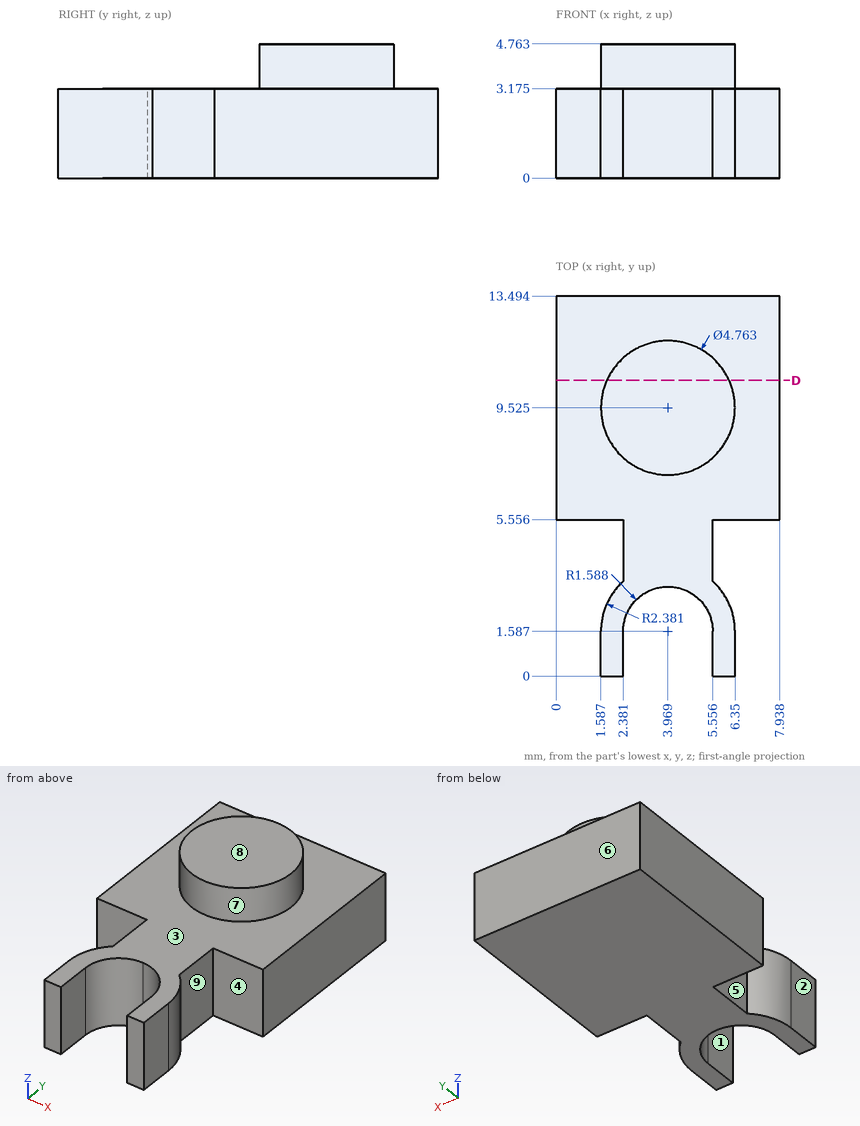
Job drawing, mm, ordinate dimensions from the low corner. One solid piece. A direction names the side the tool comes from. Coordinates: 2 decimals unless noted, no trailing zeros. Order: outer loops, then holes, each group sorted by start corner. A loop starts at its lowest first (then second) coordinate and runs counter-clockwise, first axis right, second up. Notation, with made-up numbers: (71.5, 60) - (95.5, 60) arc R21 ccw to (95.5, 91) - close; hole circle Ø4 at (4.5, -34.5). An arc over 180 degrees is marked (long way). Use CSV: the item, a comma, the result in double quotes.
Item 1: Saw through at D-D on y = 10.5. Give the cut face in (x, z) (1 decimal).
Solved:
outline,"(0, 0) - (7.9, 0) - (7.9, 3.2) - (6.1, 3.2) - (6.1, 4.8) - (1.8, 4.8) - (1.8, 3.2) - (0, 3.2) - close"
Item 2: Mould opens along Y. For the marked faces 6, 7, 8 and 9 say: +Y half, -Y half, draft (parallel to the pull), parting line (faces both ways), or undercut.
Solved:
face 6,"+Y half"
face 7,"parting line"
face 8,"draft"
face 9,"undercut"
Item 3: Probe probe 1 along X at (y, z) = (1, 2.7); probe 2 along Y at (x, z) = (5.75, 1.25) (1 decimal); probe 3 along X at (y, z) = (4.25, 0.25). List the from-to ranges inside material, lowest first.
Solved:
probe 1,"x = 1.59 to 2.38, 5.56 to 6.35"
probe 2,"y = 0 to 3.2, 5.6 to 13.5"
probe 3,"x = 2.38 to 5.56"
Item 4: 3-axis set-ups, long thin cutter, end or side, ignore diameter. For the marked faces 1, 2, 3, 4 and 5: which of +Z, -Z, +X, -X, +Y, -Y reach the whole face in a straight line?
Solved:
face 1,"+Z, -Z, -Y"
face 2,"+Z, -Z, -X, -Y"
face 3,"+Z"
face 4,"+Z, -Z, +X"
face 5,"+Z, -Z, -X"
Item 5: Drop flat-ended pins along their axis: P1, Ø2, axis at x = 7, y = 8, coming from the -Z side; P2, Ø0.8, axis at y = 1, z = 1, coming from the +X side; P3, Ø0.8, axis at y = 1, z = 1, coming from the -X side; P4, Ø0.7, axis at y = 4.5, z = 1.5, coming from the -X side. Give the stop position or say it passes through.
Solved:
P1,"stops at z = 0"
P2,"stops at x = 6.35"
P3,"stops at x = 1.59"
P4,"stops at x = 2.38"
